from build123d import *

# Parameters (mm, degrees)
SKETCH1_W           = 37
SKETCH1_H           = 37
BOSS_EXTRUDE1_DEPTH = 25
SKETCH2_W           = 28
SKETCH2_H           = 28
CUT_EXTRUDE1_DEPTH  = 37.187014245
SKETCH6_R           = 1.5
CUT_EXTRUDE3_DEPTH  = 37.187014245


with BuildPart() as part:
    # Sketch1 → Boss-Extrude1 (new body)
    with BuildSketch(Plane.XY):
        Rectangle(SKETCH1_W, SKETCH1_H)
    extrude(amount=BOSS_EXTRUDE1_DEPTH)

    # Sketch2 → Cut-Extrude1 (cut, through all)
    with BuildSketch(Plane.XY.offset(25)):
        Rectangle(SKETCH2_W, SKETCH2_H)
    extrude(amount=-CUT_EXTRUDE1_DEPTH, mode=Mode.SUBTRACT)

    # Sketch6 → Cut-Extrude3 (cut, through all)
    with BuildSketch(Plane.XY.offset(25)):
        with Locations((-16.003913062, 16.003913062)):
            Circle(SKETCH6_R)
        with Locations((16.027281765, 15.994713508)):
            Circle(SKETCH6_R)
        with Locations((16.003485412, -15.997947579)):
            Circle(SKETCH6_R)
        with Locations((-15.978784004, -16.00393382)):
            Circle(SKETCH6_R)
    extrude(amount=-CUT_EXTRUDE3_DEPTH, mode=Mode.SUBTRACT)


solid = part.part
Work out the finished part from the listing and answer in its coordinate system (mm). A direction names the side the tool comes from. Give positions to 0.01 mm unless a question says otherwise; leave off trailing zeros. Loops run counter-clockwise (first coordinate to the right, second up) from the corner with the lowest first, then second, coordinate; pieces in that order, holes last. Notation, with made-up numbers: M 15.25,71 L 59.25,71 A16 cw 59.25,96 Z; hole C 49.5,-26.5 d4. An arc over 180 degrees is marked long. Use CSV: the item, a comma, the result in double quotes.
1) Find section A-A on y = 13.5. Write down the section's boundary in (x, z).
Answer:
outline,"M -18.5,0 L -14,0 L -14,25 L -18.5,25 Z; M 14,0 L 18.5,0 L 18.5,25 L 14,25 Z"
2) Which of the six approach directions +Z, -Z, +X, -X, +Y, -Y give full straight-line access (tool end or side, diameter ignored) to faces 5 (the flat face through (18.5, 0, 12)), 6 (the flat face through (-14, 0, 13))?
Answer:
face 5,"+Z, -Z, +X, +Y, -Y"
face 6,"+Z, -Z"
3) Consider L1, parallel to X at y = 13.5, z = 2; L2, parallel to X at y = -16, z = 13. Determine where each line is inside the solid, lowest interval first.
Answer:
L1,"-18.5 to -14, 14 to 18.5"
L2,"-18.5 to -17.48, -14.48 to 14.5, 17.5 to 18.5"
4) Find section B-B on x = 16. Write down the section's boundary in (y, z), plus the area to 3 significant figures.
Answer:
outline,"M -18.5,0 L -17.5,0 L -17.5,25 L -18.5,25 Z; M -14.5,0 L 14.49,0 L 14.49,25 L -14.5,25 Z; M 17.49,0 L 18.5,0 L 18.5,25 L 17.49,25 Z"
area,"775 mm^2"
5) Find section D-D on z = 21.5. Write down the section's boundary in (x, y).
Answer:
outline,"M -18.5,-18.5 L 18.5,-18.5 L 18.5,18.5 L -18.5,18.5 Z; hole C -16,16 d3; hole C -15.98,-16 d3; hole M -14,-14 L 14,-14 L 14,14 L -14,14 Z; hole C 16,-16 d3; hole C 16.03,15.99 d3"
6) Determine the mould class of faces 1 (the cylindrical face through (-17.477, -15.938, 12.675)), 2 (the flat face through (0, -18.5, 12)), 3 (the flat face through (-15, -1, 25)), 4 (the flat face through (0, 18.5, 12)) for opening direction Y: released by +Y, released by -Y, zero draft, split by the parting line, or undercut.
Answer:
face 1,"undercut"
face 2,"released by -Y"
face 3,"zero draft"
face 4,"released by +Y"
